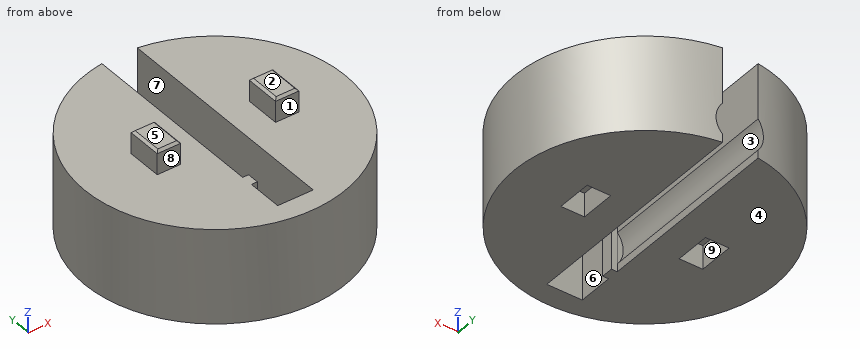
```python
from build123d import *

# Parameters (mm, degrees)
BOSS_EXTRUDE1_DEPTH             = 8
SKETCH8_R                       = 2
PIN_HOLE_DEPTH                  = 5.183346
PIN_HOLE_DIRECTION_2_REACH      = 19.493
PIN_HOLE_DIRECTION_2_END_RADIUS = 11
SKETCH6_W                       = 2
SKETCH6_H                       = 3
CUT_EXTRUDE2_DEPTH              = 2
SKETCH7_W                       = 1.98
SKETCH7_H                       = 2.98
BOSS_EXTRUDE4_DEPTH             = 1.98
CHAMFER1_SIZE                   = 0.2


with BuildPart() as part:
    # Sketch1 → Boss-Extrude1 (new body)
    with BuildSketch(Plane.XY):
        with BuildLine():
            ThreePointArc((-1.5, 10.897247359), (0, -11), (1.5, 10.897247359))
            Line((1.5, 10.897247359), (1.5, -9.183346174))
            Line((1.5, -9.183346174), (-1.5, -9.183346174))
            Line((-1.5, -9.183346174), (-1.5, -6.183346174))
            Line((-1.5, -6.183346174), (-1, -6.183346174))
            Line((-1, -6.183346174), (-1, -5.183346174))
            Line((-1, -5.183346174), (-1.5, -5.183346174))
            Line((-1.5, -5.183346174), (-1.5, 10.897247359))
        make_face()
    extrude(amount=BOSS_EXTRUDE1_DEPTH)

    # Sketch8 → pin hole (cut)
    with BuildSketch(Plane(origin=(0, 0, 0), x_dir=(1, 0, 0), z_dir=(0, 1, 0))):
        with Locations((0, -2)):
            Circle(SKETCH8_R)
    extrude(amount=-PIN_HOLE_DEPTH, mode=Mode.SUBTRACT)

    # pin hole direction 2: up to this cylinder (the profile starts inside it)
    pin_hole_direction_2_end = Plane(origin=(0, 0, 2), z_dir=(0, 0, -1)) * Cylinder(PIN_HOLE_DIRECTION_2_END_RADIUS, 61.986, mode=Mode.PRIVATE)
    # Sketch8 → pin hole direction 2 (cut, up to the surface)
    with BuildSketch(Plane(origin=(0, 0, 0), x_dir=(1, 0, 0), z_dir=(0, 1, 0)), mode=Mode.PRIVATE) as pin_hole_direction_2_sk1:
        with Locations((0, -2)):
            Circle(SKETCH8_R)
    pin_hole_direction_2_tool1 = extrude(pin_hole_direction_2_sk1.sketch, amount=PIN_HOLE_DIRECTION_2_REACH, mode=Mode.PRIVATE) & pin_hole_direction_2_end
    add(pin_hole_direction_2_tool1.solids().sort_by_distance((0, 0, 2))[0], mode=Mode.SUBTRACT)

    # Sketch6 → Cut-Extrude2 (cut)
    with BuildSketch(Plane(origin=(0, 0, 0), x_dir=(-1, 0, 0), z_dir=(0, 0, -1))):
        with Locations((-5, 0)):
            Rectangle(SKETCH6_W, SKETCH6_H)
        with Locations((5, 0)):
            Rectangle(SKETCH6_W, SKETCH6_H)
    extrude(amount=-CUT_EXTRUDE2_DEPTH, mode=Mode.SUBTRACT)

    # Sketch7 → Boss-Extrude4 (add)
    with BuildSketch(Plane.XY.offset(8)):
        with Locations((-5, 0)):
            Rectangle(SKETCH7_W, SKETCH7_H)
        with Locations((5, 0)):
            Rectangle(SKETCH7_W, SKETCH7_H)
    extrude(amount=BOSS_EXTRUDE4_DEPTH)

    # Chamfer1
    chamfer1_edges = [part.edges().sort_by_distance(p)[0] for p in [
        (-5.99, 0, 9.98),
        (-5, -1.49, 9.98),
        (-4.01, 0, 9.98),
        (-5, 1.49, 9.98),
        (4.01, 0, 9.98),
        (5, -1.49, 9.98),
        (5.99, 0, 9.98),
        (5, 1.49, 9.98),
    ]]
    chamfer(chamfer1_edges, length=CHAMFER1_SIZE)


solid = part.part
```
Part model, mm, in its own coordinate system. Face numbers are marked on the shaded views. A direction names the side the tool comes from. Round coordinates to 2 decimals unless told otherwise and drop trailing zeros. Order: outer loops, then holes, each group sorted by start corner. A loop starts at its lowest first (then second) coordinate and runs counter-clockwise, first axis right, second up. Notation, with made-up numbers: M 60.5,30 L 118.5,30 A9 cw 118.5,47 Z; hole C 58.5,-40 d6. An arc over 180 degrees is marked long. Answer in a Markdown table with one row per item. Add a question column.
Q1. Cut at B-B on z = 8.75. Give the cut face in (x, y).
Q2. Wall check: L1, parallel to Z at x = -5, y = -7; L2, parallel to X at y = 8.75, z = 4; L3, parallel to X at y = -0.75, z = 7.5. Give the ranges that are in metal, low to high. Write a range as from..to.
Q3. Pin check, flat tips, straight feed: pin 1 (2.5 mm diameter, centred on y = -8, z = 4, fed in from +X); pin 2 (5 mm diameter, centred on y = -5.5, z = 2.5, fed in from -X); pin 3 (5 mm diameter, centred on y = 4.5, z = 5, fed in from -X). Stop position of each tip, or through.
Q4. Cut at C-C on x = 0. Give the cut face in (y, z), and give its area (3 significant figures).
Q5. 3-axis set-ups, long thin cutter, end or side, ignore diameter. For the marked faces 5, 6, 7, 8 and 9: which of +Z, -Z, +X, -X, +Y, -Y reach the whole face in a straight line?
Q6. Mould opens along Z. For the marked faces 1, 2, 3 and 4 say: +Z half, -Z half, draft (parallel to the pull), parting line (faces both ways), or undercut.
Q7. Cut at D-D on y = -7.5. Give the cut face in (x, z), and give its area (3 significant figures).
Established:
| question | item | result |
|---|---|---|
| 1 | outline | M -5.99,-1.49 L -4.01,-1.49 L -4.01,1.49 L -5.99,1.49 Z; M 4.01,-1.49 L 5.99,-1.49 L 5.99,1.49 L 4.01,1.49 Z |
| 2 | L1 | z = 0..8 |
| 2 | L2 | x = -6.67..-1.5, 1.5..6.67 |
| 2 | L3 | x = -10.97..-1.5, 1.5..10.97 |
| 3 | pin 1 | stops at x = 8.69 |
| 3 | pin 2 | stops at x = -10.58 |
| 3 | pin 3 | stops at x = -10.82 |
| 4 | outline | M -11,0 L -9.18,0 L -9.18,8 L -11,8 Z |
| 4 | area | 14.5 mm2 |
| 5 | face 5 | +Z, +X, -X, +Y, -Y |
| 5 | face 6 | +Z, -Z |
| 5 | face 7 | +Z, -Z, +Y |
| 5 | face 8 | +Z, +X, -X, -Y |
| 5 | face 9 | -Z |
| 6 | face 1 | draft |
| 6 | face 2 | +Z half |
| 6 | face 3 | undercut |
| 6 | face 4 | -Z half |
| 7 | outline | M -8.05,0 L -1.5,0 L -1.5,8 L -8.05,8 Z; M 1.5,0 L 8.05,0 L 8.05,8 L 1.5,8 Z |
| 7 | area | 105 mm2 |
